Geometry: final body of the model. Coordinates: model frame, mm. Round coordinates to 2 decimals unless told otherwise and drop trailing zeros. Loops run counter-clockwise (first coordinate to the right, second up) from the corner with the lowest first, then second, coordinate; pieces in that order, holes last. Notation, with made-up numbers: M -19,13.25 L 4,13.25 A10 ccw 4,19.25 Z; hole C 85,63.5 d4. An arc over 180 degrees is marked long. Answer as a JSON object with one key per item and string values.
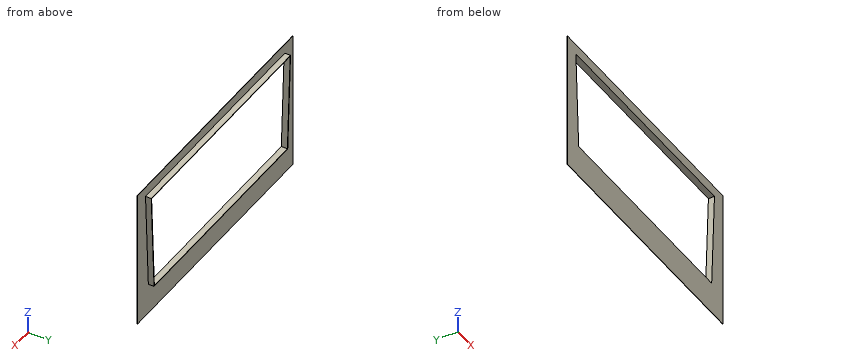
```python
from build123d import *

# Parameters (mm, degrees)
F0_W     = 2237
F0_H     = 1230
F1_DEPTH = 3
F3_DEPTH = 3.001
F5_DEPTH = 50


with BuildPart() as f1:
    # F0 (on Front) → F1 (new body)
    with BuildSketch(Plane.XZ):
        Rectangle(F0_W, F0_H)
    extrude(amount=F1_DEPTH)

    # F2 (on face) → F3 (cut, through all)
    with BuildSketch(Plane.XZ.offset(3)):
        Polygon((958.5, -335), (998.5, 525), (-998.5, 525), (-958.5, -335), (0, -335), align=None)
    extrude(amount=-F3_DEPTH, mode=Mode.SUBTRACT)

    # F4 (on face) → F5 (join)
    with BuildSketch(Plane(origin=(0, 0, 0), x_dir=(-1, 0, 0), z_dir=(0, 1, 0))):
        Polygon((1003.737964, 530), (-1003.737964, 530), (-963.272847, -340), (963.272847, -340), align=None)
        Polygon((-998.5, 525), (998.5, 525), (958.5, -335), (-958.5, -335), align=None, mode=Mode.SUBTRACT)
    extrude(amount=F5_DEPTH)


solid = f1.part
```
1) Cut plane A-A on y = 26. Return the cut outline in (x, z).
Geometry results:
{"outline": "M -1003.74,530 L -963.27,-340 L 963.27,-340 L 1003.74,530 Z; hole M -998.5,525 L -958.5,-335 L 958.5,-335 L 998.5,525 Z"}
2) First-contact query: pin 1 (6 mm diameter, centred on y = 18, z = 76.5, fed in from -X); pin 2 (10 mm diameter, centred on x = 3.5, y = 44, fed in from -Z); pin 3 (3 mm diameter, centred on x = -173, z = -350, fed in from +Y). Flat tips, straight axial feed; report the tip coordinate or a pass-through.
Geometry results:
{"pin 1": "x = -982.78", "pin 2": "z = -340", "pin 3": "y = 0"}
3) Line query: probe 1 along Z at (x, y) = (673.5, 20); probe 2 along Z at (x, y) = (-451.5, -0.5); probe 3 along Y at (x, z) = (296, -553). Output: solid intervals per line, ascending.
Geometry results:
{"probe 1": "-340 to -335, 525 to 530", "probe 2": "-615 to -335, 525 to 615", "probe 3": "-3 to 0"}
4) Cut plane B-B on x = -147. Return the cut outline in (y, z), and give its area (3 significant figures).
Geometry results:
{"outline": "M -3,-615 L 0,-615 L 0,-340 L 50,-340 L 50,-335 L -3,-335 Z; M -3,525 L 50,525 L 50,530 L 0,530 L 0,615 L -3,615 Z", "area": "1,610 mm2"}
5) Cut plane C-C on z = -59.5. Return the cut outline in (x, y).
Geometry results:
{"outline": "M -1118.5,-3 L -971.31,-3 L -971.31,50 L -976.32,50 L -976.32,0 L -1118.5,0 Z; M 971.31,-3 L 1118.5,-3 L 1118.5,0 L 976.32,0 L 976.32,50 L 971.31,50 Z"}
6) Cut plane D-D on z = -386. Return the cut outline in (x, y).
Geometry results:
{"outline": "M -1118.5,-3 L 1118.5,-3 L 1118.5,0 L -1118.5,0 Z"}
